Geometry: final body of the model. Coordinates: model frame, mm. A direction names the side the tool comes from. Give positions to 0.01 mm unless a question says otherwise; leave off trailing zeros. Write each loop counter-clockwise with the first axis right and the second up, starting at its lowest first coordinate (ties: lowest second). Pieces come first, ordered by that corner, then holes. Notation, with made-up numbers: M 41.25,18.5 L 47.25,18.5 A18 cw 47.25,35.5 Z; hole C 82,34 d10. An arc over 180 degrees is marked long. Use a Markdown table: item, result. Add a question column.
(1) Draft query along X for faces 1 (the cylindrical face through (-0.065, 5.496, -0.986)), 2 (the flat face through (1.42, -3.92, 0)), 3 (the cylindrical face through (6, 0, -1)). Return one class per face: released by +X, released by -X, zero draft, split by the parting line, or undercut.
(2) Cut plane B-B (y = 0). Output: boundary loops of the cut face in (x, z).
(3) Cut plane D-D (y = -5). Output: boundary loops of the cut face in (x, z), plus the area to 3 significant figures.
(4) Cut plane A-A (x = 0). Output: boundary loops of the cut face in (y, z), plus the area to 3 significant figures.
(5) Cut plane C-C (z = -1). Output: boundary loops of the cut face in (x, y).
(6) Pin query (flat end, axial travel): pin 1 Ø2 at (x, z) = (2, 0.5) entering from -Y; pin 2 Ø2 at (y, z) = (3.5, 0) entering from -X. Return the tip coordinate at first contact, or that it passes through.
(7) Reachability of faces 4 (the cylindrical face through (-0.867, -3.905, 1.232)), 5 (the flat face through (0, 0, -2)) from +Z, -Z, +X, -X, +Y, -Y: full face, straight path, thin tool, end or side. Return the list, or none.
(8) Material intervals for L1, parallel to Y at x = 0, z = -0.7; L2, parallel to Y at x = 0, z = 1.75; L3, parallel to Z at x = -2, y = 0.5, sorted ascending.
```python
from build123d import *

# Parameters (mm, degrees)
SKETCH1_R           = 4
SKETCH1_R_2         = 3
BOSS_EXTRUDE1_DEPTH = 3.5
CHAMFER1_SIZE       = 1
CHAMFER1_SIZE2      = 0.577350269
SKETCH2_R           = 6
BOSS_EXTRUDE2_DEPTH = 2
SKETCH3_R           = 0.5
CUT_EXTRUDE1_DEPTH  = 2


with BuildPart() as part:
    # Sketch1 → Boss-Extrude1 (new body)
    with BuildSketch(Plane.XY):
        Circle(SKETCH1_R)
        Circle(SKETCH1_R_2, mode=Mode.SUBTRACT)
    extrude(amount=BOSS_EXTRUDE1_DEPTH)

    # Chamfer1
    chamfer1_edges = [part.edges().sort_by_distance(p)[0] for p in [
        (-4, 0, 3.5),
    ]]
    chamfer1_side = [part.faces().sort_by_distance(p)[0] for p in [
        (-4, 0, 1.75),
    ]]
    chamfer(chamfer1_edges, length=CHAMFER1_SIZE, length2=CHAMFER1_SIZE2, reference=chamfer1_side[0])

    # Sketch2 → Boss-Extrude2 (add)
    with BuildSketch(Plane(origin=(0, 0, 0), x_dir=(-1, 0, 0), z_dir=(0, 0, -1))):
        Circle(SKETCH2_R)
    extrude(amount=BOSS_EXTRUDE2_DEPTH)

    # Sketch3 → Cut-Extrude1 (cut)
    with BuildSketch(Plane.XY):
        with Locations((0, 5)):
            Circle(SKETCH3_R)
        with Locations((0, -5)):
            Circle(SKETCH3_R)
    extrude(amount=-CUT_EXTRUDE1_DEPTH, mode=Mode.SUBTRACT)


solid = part.part
```
Answer list:
| question | item | result |
|---|---|---|
| 1 | face 1 | undercut |
| 1 | face 2 | zero draft |
| 1 | face 3 | split by the parting line |
| 2 | outline | M -6,-2 L 6,-2 L 6,0 L 4,0 L 4,2.5 L 3.42,3.5 L 3,3.5 L 3,0 L -3,0 L -3,3.5 L -3.42,3.5 L -4,2.5 L -4,0 L -6,0 Z |
| 3 | outline | M -3.32,-2 L -0.5,-2 L -0.5,0 L -3.32,0 Z; M 0.5,-2 L 3.32,-2 L 3.32,0 L 0.5,0 Z |
| 3 | area | 11.3 mm² |
| 4 | outline | M -6,-2 L -5.5,-2 L -5.5,0 L -6,0 Z; M -4.5,-2 L 4.5,-2 L 4.5,0 L 4,0 L 4,2.5 L 3.42,3.5 L 3,3.5 L 3,0 L -3,0 L -3,3.5 L -3.42,3.5 L -4,2.5 L -4,0 L -4.5,0 Z; M 5.5,-2 L 6,-2 L 6,0 L 5.5,0 Z |
| 4 | area | 26.4 mm² |
| 5 | outline | C 0,0 d12; hole C 0,-5 d1; hole C 0,5 d1 |
| 6 | pin 1 | y = -5.89 |
| 6 | pin 2 | x = -5.45 |
| 7 | face 4 | +Z |
| 7 | face 5 | -Z, +X, -X, +Y, -Y |
| 8 | L1 | -6 to -5.5, -4.5 to 4.5, 5.5 to 6 |
| 8 | L2 | -4 to -3, 3 to 4 |
| 8 | L3 | -2 to 0 |
